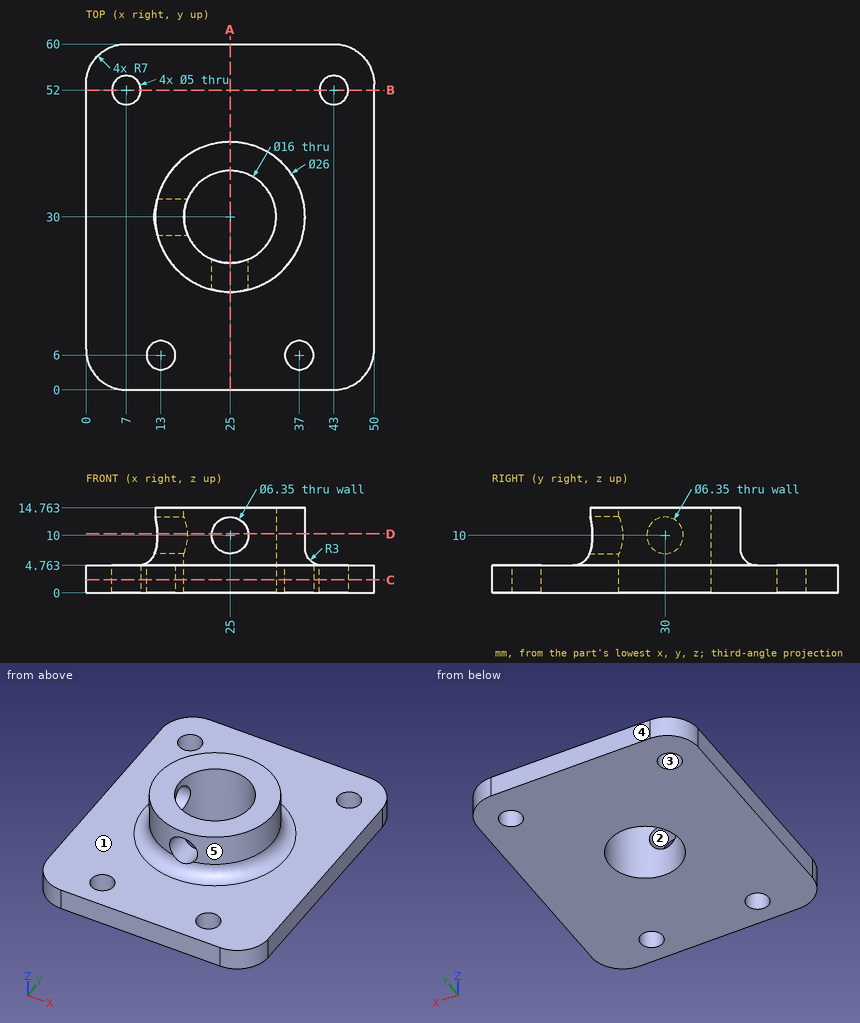
Geometry: see drawing. Coordinates: mm, zero at the bounding-box minimum. A direction names the side the tool comes from. Give positions to 0.01 mm unless a question says otherwise; leave off trailing zeros. Write each loop counter-clockwise with the first axis right and the second up, starting at its lowest first coordinate (ties: lowest second). Pieces come first, ordered by that corner, then holes. Notation, with made-up numbers: M -1.5,37.25 L 5.5,37.25 A20 ccw 5.5,62.25 Z; hole C 69,85 d9. An arc over 180 degrees is marked long. Answer in a Markdown table with one row per item. Add a question column.
(1) First-contact query: pin 1 (4 mm diameter, centred on y = 30, z = 10, fed in from -X); pin 2 (8 mm diameter, centred on x = 36.5, z = 10, fed in from +Y); pin 3 (4 mm diameter, centred on x = 25, z = 10, fed in from +Y). Flat tips, straight axial feed; report the tip coordinate or a pass-through.
(2) Section B-B on y = 52. Return loops of the section in (x, z).
(3) Section A-A on x = 25. State how many separate pieces and enclosed holes the cut face has.
(4) Ray query, line 1 (Y direction, x = 7, z = 3.3); line 2 (Y direction, x = 37, z = 3.3); line 3 (Z direction, x = 25, y = 18) (1 decimal). Return the intervals inside material, ascending.
(5) Reachability of the marked faces 4 and 5 from +Z, -Z, +X, -X, +Y, -Y: full face, straight path, thin tool, end or side. Return the list, or none.
(6) Section D-D on z = 10.25. Return loops of the section in (x, y) (1 decimal).
(7) Section C-C on z = 2.25. Return loops of the section in (x, y), and give its area (3 significant figures).
(8) Mould query, pull axis Z, two halves, no side actions, for the marked faces 1, 2 and 3. Classes: +Z half, -Z half, draft (parallel to the pull), parting line (faces both ways), or undercut.
Result set:
| question | item | result |
|---|---|---|
| 1 | pin 1 | stops at x = 32.75 |
| 1 | pin 2 | stops at y = 40.62 |
| 1 | pin 3 | stops at y = 43 |
| 2 | outline | M 0,0 L 4.5,0 L 4.5,4.76 L 0,4.76 Z; M 9.5,0 L 40.5,0 L 40.5,4.76 L 9.5,4.76 Z; M 45.5,0 L 50,0 L 50,4.76 L 45.5,4.76 Z |
| 3 | separate pieces | 3 |
| 3 | enclosed holes | 0 |
| 4 | line 1 | y = 0 to 49.5, 54.5 to 60 |
| 4 | line 2 | y = 0 to 3.5, 8.5 to 60 |
| 4 | line 3 | z = 0 to 6.8, 13.2 to 14.8 |
| 5 | face 4 | +Z, -Z, +X, -X, +Y |
| 5 | face 5 | +Z |
| 6 | outline | M 12.4,26.8 A13 ccw 21.8,17.4 L 21.8,22.7 A8 cw 17.7,26.8 Z; M 12.4,33.2 L 17.7,33.2 A8 cw long 28.2,22.7 L 28.2,17.4 A13 ccw long Z |
| 7 | outline | M 0,7 A7 ccw 7,0 L 43,0 A7 ccw 50,7 L 50,53 A7 ccw 43,60 L 7,60 A7 ccw 0,53 Z; hole C 7,52 d5; hole C 13,6 d5; hole C 25,30 d16; hole C 37,6 d5; hole C 43,52 d5 |
| 7 | area | 2,680 mm^2 |
| 8 | face 1 | +Z half |
| 8 | face 2 | undercut |
| 8 | face 3 | draft |
